Check sheet for the modelled part. Datum: model origin and axes. Units: mm. A direction names the side the tool comes from. Coordinates: 2 decimals unless noted, no trailing zeros. Loops run counter-clockwise (first coordinate to the right, second up) from the corner with the lowest first, then second, coordinate; pieces in that order, holes last. Notation, with made-up numbers: (-11, 10.5) - (30, 10.5) arc R21 cw to (30, 28.5) - close; hole circle Ø3 at (-26.5, 83.5). An arc over 180 degrees is marked (long way). Write each question's results on one line, items separated by ' | '. Start each with the question number.
1. Cross-section at D-D (z = 2.5). Record the cut outline in (x, y) (3 decimals), and give its area (3 significant figures).
2. Cross-section at A-A (y = 0). Record the cut outline in (x, z) (1 decimal).
3. Tool access check on faces 4 (the face through (9.5, -4.9, 0.2)), 5 (the face through (17.145, -2, 5)). Record the directions out of +Z, -Z, +X, -X, +Y, -Y that give a thin tool (end or side, any length) a straight path to the whole face; none if there is none.
4. Cross-section at C-C (x = 10.5). Record the cut outline in (y, z), and give its area (3 significant figures).
5. Thickness scan on line 1 (Z direction, x = 15.25, y = -3.5); line 2 (X direction, y = 2.5, z = 3); line 3 (X direction, y = 0, z = 5.05) (1 decimal). Record the ranges inside material, lowest first. Write a range as [from, to].
6. Draft check along Y on faces 1 (the face through (0, 3, 1)), 2 (the face through (7.055, 2.172, 4.965)), 3 (the face through (8.45, 3.32, 5.22)). Enter one of: released by +Y, released by -Y, zero draft, split by the parting line, or undercut.
7. Gauge pin test, flat ends, axial feed: P1, Ø4, axis at x = 9.42, y = 0, coming from the +Z side; P2, Ø2, axis at x = 9.5, z = 5, coming from the +Y side; P3, Ø5, axis at y = 0.5, z = -3, coming from the +X side (3 decimals); P4, Ø5, axis at x = 9, y = -4, coming from the +Z side. Record the tip position at first contact, or that the pin passes through.
8. Cross-section at B-B (z = -0.5). Record the cut outline in (x, y) (3 decimals), and give its area (3 significant figures).
```python
from build123d import *

# Parameters (mm, degrees)
F0_R     = 6.1849
F0_R_2   = 4.9022
F0_R_3   = 3.0099
F1_DEPTH = 2.1082
F2_DEPTH = 17.145
F3_R     = 3.2131
F4_DEPTH = 12.7


with BuildPart() as f1:
    # F0 (on Right) → F1 (new body)
    with BuildSketch(Plane.YZ):
        Circle(F0_R)
        Circle(F0_R_2, mode=Mode.SUBTRACT)
        Circle(F0_R_2)
        Circle(F0_R_3, mode=Mode.SUBTRACT)
    extrude(amount=F1_DEPTH)

    # F0 (on Right) → F2 (join)
    with BuildSketch(Plane.YZ):
        Circle(F0_R)
        Circle(F0_R_2, mode=Mode.SUBTRACT)
    extrude(amount=F2_DEPTH)

    # F3 (on Top) → F4 (cut, symmetric)
    with BuildSketch(Plane.XY):
        with Locations((9.4234, 0)):
            Circle(F3_R)
    extrude(amount=F4_DEPTH, both=True, mode=Mode.SUBTRACT)


solid = f1.part
```
Established:
1) outline: (0, -5.657) - (17.145, -5.657) - (17.145, -4.217) - (2.108, -4.217) - (2.108, -1.676) - (0, -1.676) - close; (0, 1.676) - (2.108, 1.676) - (2.108, 4.217) - (17.145, 4.217) - (17.145, 5.657) - (0, 5.657) - close | area: 60.1 mm^2
2) outline: (0, -6.2) - (6.2, -6.2) - (6.2, -4.9) - (2.1, -4.9) - (2.1, -3) - (0, -3) - close; (0, 3) - (2.1, 3) - (2.1, 4.9) - (6.2, 4.9) - (6.2, 6.2) - (0, 6.2) - close; (12.6, -6.2) - (17.1, -6.2) - (17.1, -4.9) - (12.6, -4.9) - close; (12.6, 4.9) - (17.1, 4.9) - (17.1, 6.2) - (12.6, 6.2) - close
3) face 4: +X | face 5: +Z, -Z, +X, +Y, -Y
4) outline: (-3.03, -5.39) - (-3.03, -3.86) arc R4.9 cw to (-3.03, 3.86) - (-3.03, 5.39) arc R6.18 ccw to start; (3.03, -5.39) arc R6.18 ccw to (3.03, 5.39) - (3.03, 3.86) arc R4.9 cw to (3.03, -3.86) - close | area: 28.2 mm^2
5) line 1: [-5.1, -3.43], [3.43, 5.1] | line 2: [0, 2.11] | line 3: [0, 6.2], [12.6, 17.1]
6) face 1: zero draft | face 2: undercut | face 3: split by the parting line
7) P1: through | P2: y = 4.72 | P3: x = 17.145 | P4: z = 5.74
8) outline: (0, -6.165) - (17.145, -6.165) - (17.145, -4.877) - (2.108, -4.877) - (2.108, -2.968) - (0, -2.968) - close; (0, 2.968) - (2.108, 2.968) - (2.108, 4.877) - (17.145, 4.877) - (17.145, 6.165) - (0, 6.165) - close | area: 52.2 mm^2
